from build123d import *

# Parameters (mm, degrees)
F2_W     = 100
F2_H     = 20
F3_DEPTH = 40
F6_R     = 5
F7_DEPTH = 71.0088039765
F8_R     = 5
F9_R     = 5


with BuildPart() as f1:
    # F0 (on Front) → F1 (revolve)
    with BuildSketch(Plane.XZ):
        with BuildLine():
            Line((0, 50), (0, -50))
            ThreePointArc((0, -50), (50, 0), (0, 50))
        make_face()
    revolve(axis=Axis((0, 0, -1.8287375569), (0, 0, -1)))

    # F2 (on Front) → F3 (cut, symmetric)
    with BuildSketch(Plane.XZ):
        with Locations((0, 46.6328039765)):
            Rectangle(F2_W, F2_H)
    extrude(amount=F3_DEPTH, both=True, mode=Mode.SUBTRACT)

    # F4 (on Front) → F5 (revolve, cut)
    with BuildSketch(Plane.XZ):
        with BuildLine():
            Line((0, -25), (0, -175))
            ThreePointArc((0, -175), (75, -100), (0, -25))
        make_face()
    revolve(axis=Axis((0, 0, -99.9178830534), (0, 0, -1)), mode=Mode.SUBTRACT)

    # F6 (on face) → F7 (cut, through all)
    with BuildSketch(Plane.XY.offset(36.6328039765)):
        Circle(F6_R)
    extrude(amount=-F7_DEPTH, mode=Mode.SUBTRACT)

    # F8
    f8_edges = [f1.edges().sort_by_distance(p)[0] for p in [
        (-34.029953, 0, 36.632804),
    ]]
    fillet(f8_edges, radius=F8_R)

    # F9
    f9_edges = [f1.edges().sort_by_distance(p)[0] for p in [
        (-5, 0, 36.632804),
        (-36.309219, 0, -34.375),
        (-5, 0, -25.166852),
    ]]
    fillet(f9_edges, radius=F9_R)


solid = f1.part
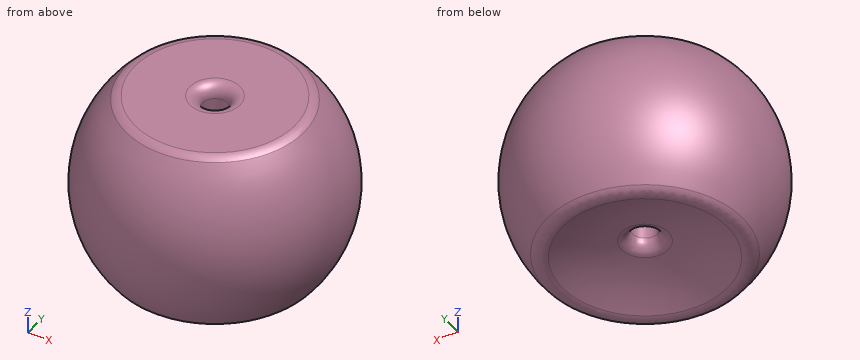
Build history of the part. All positions in model axes, mm. Give positions to 0.01 mm unless a question says otherwise; leave off trailing zeros. Order: outer loops, then holes, each group sorted by start corner. A loop starts at its lowest first (then second) coordinate and runs counter-clockwise, first axis right, second up. Notation, with made-up numbers: M -3.75,-3.75 L 51.25,-3.75 A8 ccw 51.25,2.25 Z; hole C -24.5,70 d2. An arc over 180 degrees is marked long. Use one line per item in the form item = value.
1) Drop flat-ended pins along their axis: pin 1 (3 mm diameter, centred on y = 8, z = -22.5, fed in from -X); pin 2 (3 mm diameter, centred on x = 30, z = 6, fed in from +Y); pin 3 (11.5 mm diameter, centred on x = 0, y = 0, fed in from -Z). Give the stop position or say it passes through.
Calculated:
pin_1 = -44.71
pin_2 = 40.66
pin_3 = -23.26
2) Saw through at A-A (z = -5). Give the cut face in (x, y), plus the area to 3 significant figures.
Calculated:
outline = C 0,0 d99.5; hole C 0,0 d10
area = 7,700 mm2
3) Saw through at C-C (z = -27). Give the cut face in (x, y), plus the area to 3 significant figures.
Calculated:
outline = C 0,0 d84.17; hole C 0,0 d34.41
area = 4,630 mm2
4) Saw through at B-B (x = 43.5). Give the cut face in (y, z), plus the area to 3 significant figures.
Calculated:
outline = C 0,0 d49.31
area = 1,910 mm2
5) Saw through at D-D (x = -41). Give the cut face in (y, z), plus the area to 3 significant figures.
Calculated:
outline = C 0,0 d57.24
area = 2,570 mm2
6) Probe probe 1 along Y at (x, z) = (0, 0); probe 2 along X at (y, z) = (0, 7); probe 3 along Y at (x, z) = (0, -10). List the from-to ranges inside material, lowest first.
Calculated:
probe_1 = -50 to -5, 5 to 50
probe_2 = -49.51 to -5, 5 to 49.51
probe_3 = -48.99 to -5, 5 to 48.99
